Read the model definition and answer for the solid it produces. Units are mm, in the model's axes. A direction names the side the tool comes from. Coordinates: 2 decimals unless noted, no trailing zeros. Order: outer loops, then holes, each group sorted by start corner. A loop starts at its lowest first (then second) coordinate and runs counter-clockwise, first axis right, second up. Notation, with made-up numbers: (4.25, -23) -> (33.25, -23) arc R15 cw to (33.25, -6) -> close; hole circle Ø8 at (83, 18). An arc over 180 degrees is marked (long way). Use CSV: the item, a comma, the result in double quotes.
```python
from build123d import *

# Parameters (mm, degrees)
F1_DEPTH = 7.5
F2_DEPTH = 2.5
F4_DEPTH = 25
F5_DEPTH = 3.5


with BuildPart() as f1:
    # F0 (on Top) → F1 (new body)
    with BuildSketch(Plane.XY):
        Polygon((0, -20), (0, 0), (-20, 0), align=None)
    extrude(amount=F1_DEPTH)

    # F1_face (on face) → F2 (join)
    with BuildSketch(Plane(origin=(-6.666667, -6.666667, 0), x_dir=(1, 0, 0), z_dir=(0, 0, -1))):
        Polygon((6.666667, -6.666667), (6.666667, 13.333333), (-13.333333, -6.666667), align=None)
    extrude(amount=F2_DEPTH)

    # F3 (on face) → F4 (cut)
    with BuildSketch(Plane(origin=(0, 0, -2.5), x_dir=(1, 0, 0), z_dir=(0, 0, -1))):
        with BuildLine():
            ThreePointArc((-2, 5), (-3.85195, 7.771639), (-7.12132, 7.12132))
            ThreePointArc((-7.12132, 7.12132), (-6.14805, 2.228361), (-2, 5))
        make_face()
    extrude(amount=-F4_DEPTH, mode=Mode.SUBTRACT)

    # F3 (on face) → F5 (cut)
    with BuildSketch(Plane(origin=(0, 0, -2.5), x_dir=(1, 0, 0), z_dir=(0, 0, -1))):
        Polygon((-3.77061, 9.588148), (-8.358757, 8.358757), (-9.588148, 3.77061), (-6.22939, 0.411852), (-1.641243, 1.641243), (-0.411852, 6.22939), align=None)
        with BuildLine():
            ThreePointArc((-2, 5), (-6.14805, 2.228361), (-7.12132, 7.12132))
            ThreePointArc((-7.12132, 7.12132), (-3.85195, 7.771639), (-2, 5))
        make_face(mode=Mode.SUBTRACT)
    extrude(amount=-F5_DEPTH, mode=Mode.SUBTRACT)


solid = f1.part
```
Item 1: Find section B-B, the plane y = -7.5. Give the vertices of the cut face in (x, z), then the cut area to 3 significant figures.
Return value:
outline,"(-12.5, -2.5) -> (-8.59, -2.5) -> (-8.59, 1) -> (-6.66, 1) -> (-6.66, 7.5) -> (-12.5, 7.5) -> close; (-3.34, 1) -> (-1.68, 1) -> (-1.68, -2.5) -> (0, -2.5) -> (0, 7.5) -> (-3.34, 7.5) -> close"
area,"79.3 mm^2"
Item 2: Straight lines are drawn through the part: line 1 along Z through (x, y) = (-5.25, -8.75); line 2 along X through (y, z) = (-5, 6.25); line 3 along X through (y, z) = (-3.5, -0.75). For each, find the intervals that lie inside material, in ascending order.
Return value:
line 1,"z = 1 to 7.5"
line 2,"x = -15 to -8, -2 to 0"
line 3,"x = -16.5 to -9.32, -1.14 to 0"
Item 3: Each of these flat-tipped pins is pushed along its axis until it touches: P1, Ø5, axis at x = -5, y = -5, coming from the -Z side; P2, Ø5, axis at x = -17, z = 2.5, coming from the +Y side; P3, Ø5, axis at x = -5, z = 6, coming from the -Y side; P4, Ø3, axis at x = -4.5, y = -6.5, coming from the -Z side. Where does it stop, or does it pass through?
Return value:
P1,"passes through"
P2,"stops at y = 0"
P3,"stops at y = -17.5"
P4,"stops at z = 1"
Item 4: A tool of negligible diameter and unlimited length cuts with its end or side. For faces 4 (the flat face through (-8.965, -6.097, -0.774)), 5 (the flat face through (0, -10, 3)), from which of +Z, -Z, +X, -X, +Y, -Y can it reach the whole face along a straight path? Write none if from no direction.
Return value:
face 4,"-Z"
face 5,"+Z, -Z, +X, +Y, -Y"
Item 5: The mould has two halves that part along X. Classify faces 1 (the flat face through (-1.035, -3.903, -0.774)), 2 (the flat face through (-10, 0, 3)), 3 (the flat face through (-10, -10, 3)): +X half, -X half, draft (parallel to the pull), parting line (faces both ways), or undercut.
Return value:
face 1,"undercut"
face 2,"draft"
face 3,"-X half"
Item 6: Find section D-D, the plane x = -9. Give the vertices of the cut face in (y, z).
Return value:
outline,"(-11, -2.5) -> (-5.97, -2.5) -> (-5.97, 1) -> (-3.18, 1) -> (-3.18, -2.5) -> (0, -2.5) -> (0, 7.5) -> (-11, 7.5) -> close"
Item 7: Find section A-A, the plane z = 5. Give the vertices of the cut face in (x, y).
Return value:
outline,"(-20, 0) -> (0, -20) -> (0, 0) -> close; hole (-7.12, -7.12) arc R3 ccw to (-2, -5) arc R3 ccw (long way) to start"
Item 8: Find section C-C, the plane x = -5. Give the vertices of the cut face in (y, z).
Return value:
outline,"(-15, -2.5) -> (-9.26, -2.5) -> (-9.26, 1) -> (-8, 1) -> (-8, 7.5) -> (-15, 7.5) -> close; (-2, 1) -> (-0.74, 1) -> (-0.74, -2.5) -> (0, -2.5) -> (0, 7.5) -> (-2, 7.5) -> close"
